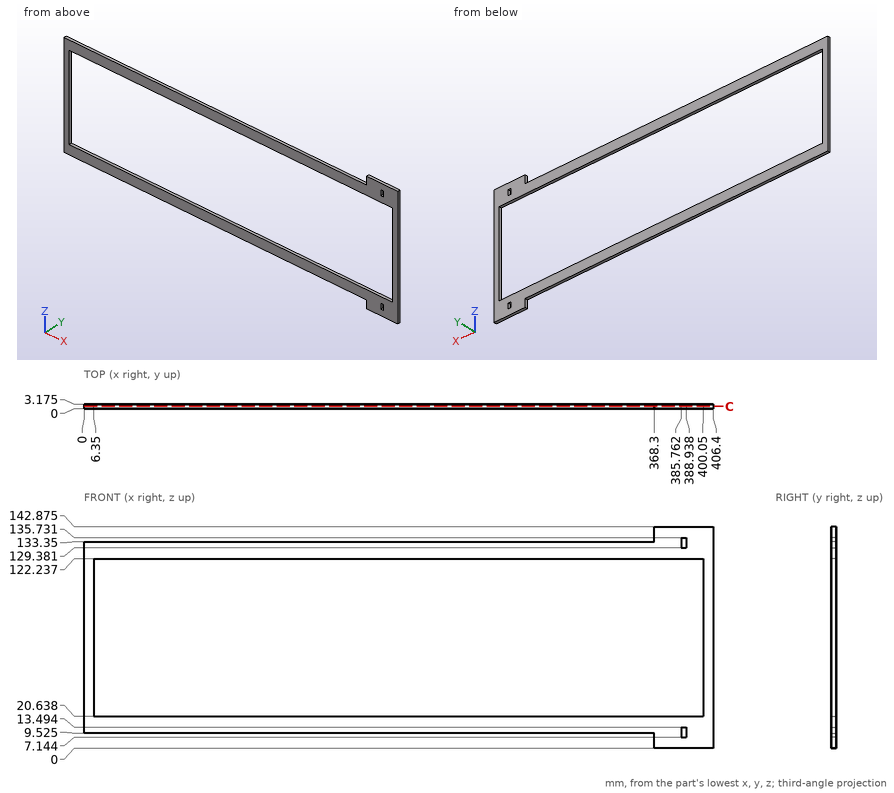
For this review, use the dimensioned drawing (mm, ordinates from the lowest corner) and the shaded views. Round coordinates to 2 decimals unless told otherwise and drop trailing zeros. Answer as CSV lines item,"result". Start each with the question number.
(1) To check wall thickness, follow line 1 (X direction, y = 0.3, z = 118); line 2 (Z direction, x = 370, y = 1.15) (1 decimal). State the ranges of each line that lie inside material, in increasing order.
(2) For pin 1 Ø1 at (y, z) = (1.5, 6.5) entering from -X; pin 2 Ø1 at (x, y) = (112.5, 1) entering from -Z (1 decimal), all flat-tipped, find the tip position at first contact; note any pin that passes through.
(3) We need section C-C on y = 1.7. Give the number of separate pieces and of enclosed holes in the cut face, plus the area to 3 significant figures.
Worked answers:
1,line 1,"0 to 6.35, 400.05 to 406.4"
1,line 2,"0 to 20.6, 122.2 to 142.9"
2,pin 1,"x = 368.3"
2,pin 2,"z = 9.5"
3,separate pieces,"1"
3,enclosed holes,"3"
3,area,"11,000 mm²"
